The listing builds one solid part. Answer for the finished solid, in the listing's coordinates (mm). A direction names the side the tool comes from. Coordinates: 2 decimals unless noted, no trailing zeros. Order: outer loops, then holes, each group sorted by start corner. A loop starts at its lowest first (then second) coordinate and runs counter-clockwise, first axis right, second up. Notation, with made-up numbers: (23, 15) - (74, 15) arc R22 cw to (74, 42) - close; hole circle Ø10 at (-27.5, -29). An arc over 180 degrees is marked (long way). Use a Markdown table: item, result. Add a question column.
Item 1: The part is cut by section D-D, the plane z = -13. Give the vertices of the cut face in (x, y).
Item 2: Flat-ended cylindrical pins translate along their axes: P1, Ø2, axis at x = 5, y = 5, coming from the -Z side; P2, Ø1.8, axis at x = 7.5, z = -14, coming from the +Y side; P3, Ø1.5, axis at x = 3, z = 3, coming from the +Y side. Find the tip coordinate at first contact, or state that the pin passes through.
Item 3: For faces 4 (the flat face through (5, -3, 12.5)), 5 (the flat face through (0, -7, 0)), determine the directions among +Z, -Z, +X, -X, +Y, -Y from which every point of the face is accessible in a straight line to the end or side of a thin tool.
Item 4: The part is cut by section C-C, the plane x = 2. Give the vertices of the cut face in (y, z), then the cut area to 3 significant figures.
Item 5: Find the intervals of material crossed by line 1 along Z through (x, y) = (8, 1.5); line 2 along Y through (x, z) = (5, 18.6); line 3 along Z through (x, y) = (8.5, -2), in increasing order.
Item 6: The part is cut by section B-B, the plane y = 5. Give the vertices of the cut face in (x, z).
Item 7: The part is cut by section A-A, the plane x = 5. Give the vertices of the cut face in (y, z).
Item 8: The mould has two halves that part along Z. Classify faces 1 (the flat face through (5, -5.5, 0)), 2 (the flat face through (5, 0, -21)), 3 (the cylindrical face through (4.15, 6.63, 18.47)): released by +Z, released by -Z, zero draft, split by the parting line, or undercut.
from build123d import *

# Parameters (mm, degrees)
SKETCH1_W               = 3.5
SKETCH1_H               = 5
BOSS_EXTRUDE1_DEPTH     = 10
CUT_EXTRUDE1_DEPTH      = 53
CUT_EXTRUDE1_DEPTH_BACK = 10
SKETCH2_R               = 1.836585915


with BuildPart() as part:
    # Sketch1 → Boss-Extrude1 (new body)
    with BuildSketch(Plane(origin=(0, 0, 0), x_dir=(0, 0, -1), z_dir=(1, 0, 0))):
        Polygon((-21, 10.5), (-21, -10.5), (21, -10.5), (21, 10.5), (16, 10.5), (16, -0.5), (16, -5.5), (12.5, -5.5), (-12.5, -5.5), (-16, -5.5), (-16, -0.5), (-16, 10.5), align=None)
        with Locations((-14.25, -3)):
            Rectangle(SKETCH1_W, SKETCH1_H)
        with Locations((14.25, -3)):
            Rectangle(SKETCH1_W, SKETCH1_H)
    extrude(amount=BOSS_EXTRUDE1_DEPTH)

    # Sketch2 → Cut-Extrude1 (cut, two sides: drawn at the far end of the back side and taken through both)
    with BuildSketch(Plane.XY.offset(-16).offset(-CUT_EXTRUDE1_DEPTH_BACK)):
        with Locations(Location((5, 5, 0), (0, 0, 180))):
            Circle(SKETCH2_R)
    extrude(amount=CUT_EXTRUDE1_DEPTH + CUT_EXTRUDE1_DEPTH_BACK, mode=Mode.SUBTRACT)


solid = part.part
Solution:
| question | item | result |
|---|---|---|
| 1 | outline | (0, -10.5) - (10, -10.5) - (10, -0.5) - (0, -0.5) - close |
| 2 | P1 | passes through |
| 2 | P2 | stops at y = -0.5 |
| 2 | P3 | stops at y = -5.5 |
| 3 | face 4 | +X, -X, +Y |
| 3 | face 5 | +Z, -Z, -X, +Y, -Y |
| 4 | outline | (-10.5, -21) - (10.5, -21) - (10.5, -16) - (-0.5, -16) - (-0.5, -12.5) - (-5.5, -12.5) - (-5.5, 12.5) - (-0.5, 12.5) - (-0.5, 16) - (10.5, 16) - (10.5, 21) - (-10.5, 21) - close |
| 4 | area | 405 mm2 |
| 5 | line 1 | z = -21 to -16, 16 to 21 |
| 5 | line 2 | y = -10.5 to 3.16, 6.84 to 10.5 |
| 5 | line 3 | z = -21 to -12.5, 12.5 to 21 |
| 6 | outline | (0, -21) - (3.16, -21) - (3.16, -16) - (0, -16) - close; (0, 16) - (3.16, 16) - (3.16, 21) - (0, 21) - close; (6.84, -21) - (10, -21) - (10, -16) - (6.84, -16) - close; (6.84, 16) - (10, 16) - (10, 21) - (6.84, 21) - close |
| 7 | outline | (-10.5, -21) - (3.16, -21) - (3.16, -16) - (-0.5, -16) - (-0.5, -12.5) - (-5.5, -12.5) - (-5.5, 12.5) - (-0.5, 12.5) - (-0.5, 16) - (3.16, 16) - (3.16, 21) - (-10.5, 21) - close; (6.84, -21) - (10.5, -21) - (10.5, -16) - (6.84, -16) - close; (6.84, 16) - (10.5, 16) - (10.5, 21) - (6.84, 21) - close |
| 8 | face 1 | undercut |
| 8 | face 2 | released by -Z |
| 8 | face 3 | zero draft |
